from build123d import *

# Parameters (mm, degrees)
SKETCH_R        = 1.8
PAD_DEPTH       = 3
POCKET_DEPTH    = 2
SKETCH002_W     = 9.3
SKETCH002_H     = 15
PAD001_DEPTH    = 15
SKETCH003_R     = 2.5
POCKET001_DEPTH = 10
FILLET_R        = 7.45
POCKET002_DEPTH = 15
FILLET001_R     = 7
FILLET002_R     = 2


with BuildPart() as part:
    # Sketch → Pad (new body)
    with BuildSketch(Plane(origin=(0, 0, 0), x_dir=(1, 0, 0), z_dir=(0, 0, -1))):
        with BuildLine():
            ThreePointArc((0, 5), (-3.535534, 3.535534), (-5, 0))
            Line((-5, 0), (-5, -29))
            ThreePointArc((-5, -29), (-3.535534, -32.535534), (0, -34))
            Line((0, -34), (30, -34))
            ThreePointArc((30, -34), (33.535534, -32.535534), (35, -29))
            Line((35, 0), (35, -29))
            ThreePointArc((35, 0), (33.535534, 3.535534), (30, 5))
            Line((0, 5), (30, 5))
        make_face()
        Circle(SKETCH_R, mode=Mode.SUBTRACT)
        with Locations((30, 0)):
            Circle(SKETCH_R, mode=Mode.SUBTRACT)
        with Locations((30, -29)):
            Circle(SKETCH_R, mode=Mode.SUBTRACT)
        with Locations((0, -29)):
            Circle(SKETCH_R, mode=Mode.SUBTRACT)
    extrude(amount=PAD_DEPTH)

    # Sketch001 → Pocket (cut)
    with BuildSketch(Plane(origin=(0, 0, -3), x_dir=(1, 0, 0), z_dir=(0, 0, -1))):
        Polygon((-3, -30.732051), (-3, -27.267949), (0, -25.535898), (3, -27.267949), (3, -30.732051), (0, -32.464102), align=None)
        Polygon((27, -30.732051), (27, -27.267949), (30, -25.535898), (33, -27.267949), (33, -30.732051), (30, -32.464102), align=None)
        Polygon((-3, 1.732051), (-3, -1.732051), (0, -3.464102), (3, -1.732051), (3, 1.732051), (0, 3.464102), align=None)
        Polygon((27, -1.732051), (27, 1.732051), (30, 3.464102), (33, 1.732051), (33, -1.732051), (30, -3.464102), align=None)
    extrude(amount=-POCKET_DEPTH, mode=Mode.SUBTRACT)

    # Sketch002 → Pad001 (new body)
    with BuildSketch(Plane(origin=(0, 0, -3), x_dir=(1, 0, 0), z_dir=(0, 0, -1))):
        with Locations((15, -14.5)):
            Rectangle(SKETCH002_W, SKETCH002_H)
    extrude(amount=PAD001_DEPTH)

    # Sketch003 → Pocket001 (cut)
    with BuildSketch(Plane(origin=(19.65, 0, 0), x_dir=(0, -1, 0), z_dir=(1, 0, 0))):
        with Locations((-14.5, 10.5)):
            Circle(SKETCH003_R)
    extrude(amount=-POCKET001_DEPTH, mode=Mode.SUBTRACT)

    # Fillet
    fillet_edges = [part.edges().sort_by_distance(p)[0] for p in [
        (15, 22, -18),
        (15, 7, -18),
    ]]
    fillet(fillet_edges, radius=FILLET_R)

    # Sketch004 → Pocket002 (cut)
    with BuildSketch(Plane(origin=(0, 22, 0), x_dir=(1, 0, 0), z_dir=(0, 1, 0))):
        Polygon((13.35, 18), (13.35, 3), (16.65, 3), (16.65, 18), (15, 18), align=None)
    extrude(amount=-POCKET002_DEPTH, mode=Mode.SUBTRACT)

    # Fillet001
    fillet001_edges = [part.edges().sort_by_distance(p)[0] for p in [
        (18.15, 22, -3),
        (11.85, 22, -3),
    ]]
    fillet(fillet001_edges, radius=FILLET001_R)

    # Fillet002
    fillet002_edges = [part.edges().sort_by_distance(p)[0] for p in [
        (18.15, 7, -3),
        (11.85, 7, -3),
    ]]
    fillet(fillet002_edges, radius=FILLET002_R)


solid = part.part
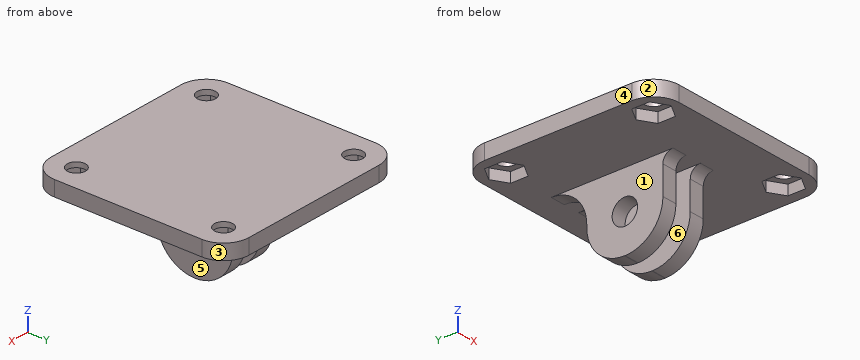
The listing builds one solid part. Answer for the finished solid, in the listing's coordinates (mm). Face numbers are marked on the shaded views. A direction names the side the tool comes from. Coordinates: 2 decimals unless noted, no trailing zeros. Order: outer loops, then holes, each group sorted by start corner. A loop starts at its lowest first (then second) coordinate and runs counter-clockwise, first axis right, second up.
Q1. A cutting plane is placed at A-A, the plane z = -1.5. State how many separate pieces and enclosed holes the cut face has, and give its area (3 significant figures).
Q2. A cutting plane is placed at C-C, the plane x = 30.5. Write down the section's boundary in (y, z).
Q3. A cutting plane is placed at B-B, the plane z = -12.25. Write down the section's boundary in (x, y), and give its area (3 significant figures).
Q4. A cutting plane is placed at D-D, the plane y = 24.5. Write down the section's boundary in (x, z).
Q5. Given P1, Ø0.6, axis at y = -0.5, z = -2, coming from the -X side; P2, Ø3, axis at x = 0, y = 29, coming from the +Z side; P3, Ø7.5, axis at y = 22.5, z = -8.5, coming from the -X side; P4, Ø10, axis at x = 5.5, z = -9.5, coming from the +Y side, each flat-ended and moving along its own axis, determine where each tip first touches the part or whether it passes through.
Q6. Consider line 1 (Y direction, x = 30, z = -0.65); line 2 (X direction, y = 0, z = -0.75); line 3 (Z direction, x = 12.05, y = 14.5). Determine where each line is inside the solid, lowest interval first.
Q7. For a pull along Y with two mould halves and no side action, classify the marked faces 1, 2 and 3 as pulls with the +Y half, pulls with the -Y half, needs draft (parallel to the pull), parting line crosses it, or undercut.
Q8. Which of the six approach directions +Z, -Z, +X, -X, +Y, -Y give full straight-line access (tool end or side, diameter ignored) to the marked faces 4, 5 and 6?
Answers follow:
1. separate pieces: 1
1. enclosed holes: 4
1. area: 1,410 mm2
2. outline: (-4.97, -3) - (-3.18, -3) - (-3.18, -1) - (-1.73, -1) - (-1.73, 0) - (-4.97, 0) - close; (1.73, -1) - (3.18, -1) - (3.18, -3) - (25.82, -3) - (25.82, -1) - (27.27, -1) - (27.27, 0) - (1.73, 0) - close; (30.73, -1) - (32.18, -1) - (32.18, -3) - (33.97, -3) - (33.97, 0) - (30.73, 0) - close
3. outline: (10.35, 7.2) - (13.35, 7.2) - (13.35, 12.71) - (10.35, 12.71) - close; (10.35, 16.29) - (13.35, 16.29) - (13.35, 21.8) - (10.35, 21.8) - close; (16.65, 7.2) - (19.65, 7.2) - (19.65, 12.71) - (16.65, 12.71) - close; (16.65, 16.29) - (19.65, 16.29) - (19.65, 21.8) - (16.65, 21.8) - close
3. area: 66.2 mm2
4. outline: (-5, -3) - (10.35, -3) - (10.35, -4.64) - (13.35, -4.64) - (13.35, -3) - (16.65, -3) - (16.65, -4.64) - (19.65, -4.64) - (19.65, -3) - (35, -3) - (35, 0) - (-5, 0) - close
5. P1: stops at x = -5
5. P2: passes through
5. P3: stops at x = 10.35
5. P4: stops at y = 22.21
6. line 1: y = -5 to -1.8, 1.8 to 27.2, 30.8 to 34
6. line 2: x = -5 to -1.8, 1.8 to 28.2, 31.8 to 35
6. line 3: z = -18 to -13, -8 to 0
7. face 1: needs draft
7. face 2: pulls with the -Y half
7. face 3: pulls with the +Y half
8. face 4: +Z, -Z, -X, +Y, -Y
8. face 5: -Z, +X, +Y, -Y
8. face 6: -Z, +Y, -Y
